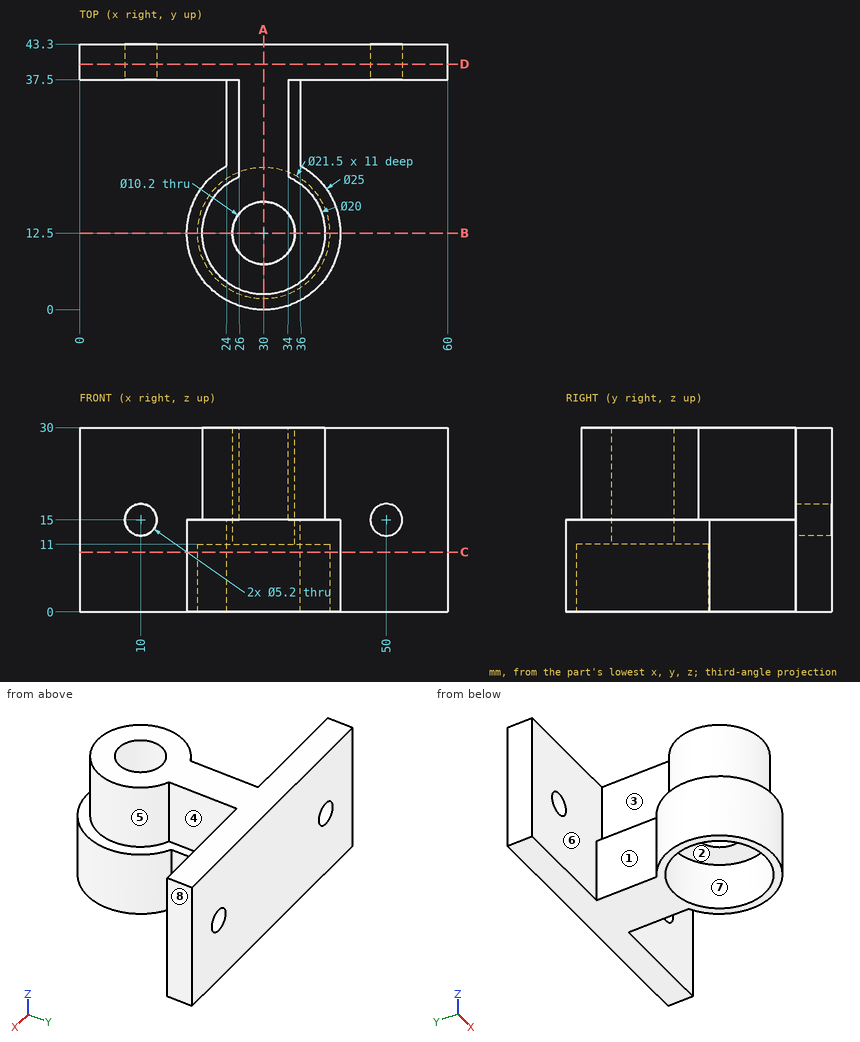
Study the drawing (mm; zero at the part's minimum x, y, z) and answer. A direction names the side the tool comes from. Give positions to 0.01 mm unless a question says otherwise; leave off trailing zeros. Order: outer loops, then holes, each group sorted by start corner. A loop starts at its lowest first (then second) coordinate and runs counter-clockwise, first axis right, second up. Notation, with made-up numbers: M 12.5,31 L 23.5,31 A12 cw 23.5,48 Z; hole C 12.5,-33.75 d9. An arc over 180 degrees is marked long. Put each result on its own line as item: value. Start each with the question number.
Item 1: For a pull along X with two mould halves and no side action, classify the marked faces 6, 7 and 8 as +X half, -X half, draft (parallel to the pull), parting line (faces both ways), or undercut.
Item 2: Find the intervals of material crossed by line 1 along X through (y, z) = (41.65, 15); line 2 along Y through (x, z) = (30, 15.5); line 3 along Y through (x, z) = (30, 8.5), in increasing order.
Item 3: The part is cut by section A-A, the plane x = 30. Determine the outline of the cut face in (y, z).
Item 4: Which of the six approach directions +Z, -Z, +X, -X, +Y, -Y give full straight-line access (tool end or side, diameter ignored) to the marked faces 1, 2, 3, 4 and 5?
Item 5: The part is cut by section C-C, the plane z = 9.75. Determine the outline of the cut face in (x, y), and give its area (3 significant figures).
Item 6: The part is cut by section D-D, the plane y = 40. Determine the outline of the cut face in (x, z), and give its area (3 significant figures).
Item 7: Flat-ended cylindrical pins translate along their axes: P1, Ø5, axis at x = 24, y = 16.5, coming from the -Z side; P2, Ø4, axis at y = 24.5, z = 23, coming from the +X side; P3, Ø10, axis at y = 7, z = 6, coming from the +X side. Find the tip coordinate at first contact, or state that the pin passes through.
Item 8: The part is cut by section B-B, the plane y = 12.5. Determine the outline of the cut face in (x, z), and give its area (3 significant figures).
Answer key:
1. face 6: draft
1. face 7: undercut
1. face 8: +X half
2. line 1: x = 0 to 7.4, 12.6 to 47.4, 52.6 to 60
2. line 2: y = 2.5 to 7.4, 17.6 to 43.3
2. line 3: y = 0 to 1.75, 23.25 to 43.3
3. outline: M 0,0 L 1.75,0 L 1.75,11 L 7.4,11 L 7.4,30 L 2.5,30 L 2.5,15 L 0,15 Z; M 17.6,11 L 23.25,11 L 23.25,0 L 43.3,0 L 43.3,30 L 17.6,30 Z
4. face 1: +Z, -Z, -X
4. face 2: -Z
4. face 3: +Z, -X
4. face 4: +Z, +X
4. face 5: +Z
5. outline: M 0,37.5 L 24,37.5 L 24,23.47 A12.5 ccw long 36,23.47 L 36,37.5 L 60,37.5 L 60,43.3 L 0,43.3 Z; hole C 30,12.5 d21.5
5. area: 632 mm²
6. outline: M 0,0 L 60,0 L 60,30 L 0,30 Z; hole C 10,15 d5.2; hole C 50,15 d5.2
6. area: 1,760 mm²
7. P1: stops at z = 11
7. P2: stops at x = 34
7. P3: stops at x = 42.49
8. outline: M 17.5,0 L 19.25,0 L 19.25,11 L 24.9,11 L 24.9,30 L 20,30 L 20,15 L 17.5,15 Z; M 35.1,11 L 40.75,11 L 40.75,0 L 42.5,0 L 42.5,15 L 40,15 L 40,30 L 35.1,30 Z
8. area: 245 mm²
